Read the model definition and answer for the solid it produces. Units are mm, in the model's axes. A direction names the side the tool comes from. Coordinates: 2 decimals unless noted, no trailing zeros. Write each loop counter-clockwise with the first axis right and the second up, starting at its lowest first coordinate (ties: lowest second). Pieces come first, ordered by that corner, then holes. Notation, with made-up numbers: M 51.25,-39.5 L 109.25,-39.5 A31 ccw 109.25,-5.5 Z; hole C 70.5,-12 d2. An arc over 180 degrees is marked long. Write item = value, one per line.
from build123d import *

# Parameters (mm, degrees)
BOSS_EXTRUDE1_DEPTH   = 180
F_6_CLEARANCE_HOLE1_D = 3.7973
F_6_CLEARANCE_HOLE2_D = 3.7973


with BuildPart() as part:
    # Sketch1 → Boss-Extrude1 (new body)
    with BuildSketch(Plane.XY):
        Polygon((0, 0), (0, 17), (-3, 17), (-3, 3), (-17, 3), (-17, 0), align=None)
    extrude(amount=BOSS_EXTRUDE1_DEPTH)

    # #6 Clearance Hole1 (through all)
    with Locations(Plane.ZY.offset(3)):
        with Locations((30, 12), (100, 12), (170, 12)):
            Hole(F_6_CLEARANCE_HOLE1_D / 2)

    # #6 Clearance Hole2 (through all)
    with Locations(Plane(origin=(0, 3, 0), x_dir=(1, 0, 0), z_dir=(0, 1, 0))):
        with Locations((-12, -20), (-12, -90), (-12, -160)):
            Hole(F_6_CLEARANCE_HOLE2_D / 2)


solid = part.part
Item 1: Consider line 1 along X through (y, z) = (1.55, 20); line 2 along Z through (x, y) = (-12, 2.2); line 3 along Y through (x, z) = (-0.85, 170). Determine where each line is inside the solid, lowest interval first. Write a range as from..to.
Worked answers:
line_1 = -17..-13.9, -10.1..0
line_2 = 0..18.1, 21.9..88.1, 91.9..158.1, 161.9..180
line_3 = 0..10.1, 13.9..17
Item 2: Find section B-B (z = 100). Determine the outline of the cut face in (x, y).
Worked answers:
outline = M -17,0 L 0,0 L 0,10.1 L -3,10.1 L -3,3 L -17,3 Z; M -3,13.9 L 0,13.9 L 0,17 L -3,17 Z
Item 3: Flat-ended cylindrical pins translate along their axes: pin 1 (6 mm diameter, centred on y = 11, z = 89.5, fed in from +X); pin 2 (4 mm diameter, centred on x = -9.5, z = 133, fed in from +Y); pin 3 (2.5 mm diameter, centred on y = 12, z = 30, fed in from -X); pin 4 (4 mm diameter, centred on y = 11, z = 127.5, fed in from -X). Find the tip coordinate at first contact, or state that the pin passes through.
Worked answers:
pin_1 = 0
pin_2 = 3
pin_3 = through
pin_4 = -3
Item 4: Find section C-C (x = -12). Determine the outline of the cut face in (y, z), and give its area (3 significant figures).
Worked answers:
outline = M 0,0 L 3,0 L 3,18.1 L 0,18.1 Z; M 0,21.9 L 3,21.9 L 3,88.1 L 0,88.1 Z; M 0,91.9 L 3,91.9 L 3,158.1 L 0,158.1 Z; M 0,161.9 L 3,161.9 L 3,180 L 0,180 Z
area = 506 mm²
Item 5: Find section A-A (y = 12). Determine the outline of the cut face in (x, z), and give its area (3 significant figures).
Worked answers:
outline = M -3,0 L 0,0 L 0,28.1 L -3,28.1 Z; M -3,31.9 L 0,31.9 L 0,98.1 L -3,98.1 Z; M -3,101.9 L 0,101.9 L 0,168.1 L -3,168.1 Z; M -3,171.9 L 0,171.9 L 0,180 L -3,180 Z
area = 506 mm²
Item 6: Find section D-D (z = 40). Determine the outline of the cut face in (x, y).
Worked answers:
outline = M -17,0 L 0,0 L 0,17 L -3,17 L -3,3 L -17,3 Z
Item 7: Which of the six approach directions +Z, -Z, +X, -X, +Y, -Y give full straight-line access (tool end or side, diameter ignored) to faces 1 (the face through (-10, 3, 89)), 2 (the face through (0, 8, 89))?
Worked answers:
face_1 = +Z, -Z, -X, +Y
face_2 = +Z, -Z, +X, +Y, -Y
Item 8: For a pull along Y with two mould halves and no side action, classify faces 3 (the face through (-1.479, 12.083, 171.897)), 4 (the face through (-1, 17, 89)), 5 (the face through (-3, 10, 89)) as released by +Y, released by -Y, zero draft, split by the parting line, or undercut.
Worked answers:
face_3 = undercut
face_4 = released by +Y
face_5 = zero draft
